Source: CAD feature listing. Evaluate the final solid. Frame: model axes, mm. Face numbers are marked on the shaded views. A direction names the side the tool comes from. Give positions to 0.01 mm unless a question says otherwise; leave off trailing zeros. Order: outer loops, then holes, each group sorted by start corner. A loop starts at its lowest first (then second) coordinate and runs counter-clockwise, first axis right, second up. Notation, with made-up numbers: M 57,-34.5 L 102,-34.5 A33 ccw 102,-3.5 Z; hole C 23,24.5 d2. An arc over 180 degrees is marked long. Answer in a Markdown table with one row per item. Add a question column.
(1) Section query A-A, the plane z = 22. Return loops of the section in (x, y).
(2) Section query C-C, the plane x = 0. Return loops of the section in (y, z), plus the area to 4 significant figures.
(3) Section query B-B, the plane z = 0. Return loops of the section in (x, y).
(4) Material intervals for line 1 along Z through (x, y) = (22, 0.65); line 2 along X through (y, z) = (7.5, 0), sorted ascending.
(5) Pin query (flat end, axial travel): P1, Ø1, axis at y = 2.5, z = -11.5, coming from the -X side; P2, Ø2, axis at y = -0.5, z = -17.5, coming from the +X side. Return the tip coordinate at first contact, or that it passes through.
(6) Section query D-D, the plane x = -22. Return loops of the section in (y, z), plus the area to 3 significant figures.
(7) Set-up query: the marked faces 1 and 2. Return all of +Z, -Z, +X, -X, +Y, -Y with unobstructed straight access to the full face (end or side cutting, diameter ignored); none if empty.
from build123d import *

# Parameters (mm, degrees)
SKETCH1_R                = 27.5
SKETCH1_R_2              = 12.5
SKETCH1_R_3              = 1
BOSS_EXTRUDE1_DEPTH      = 1.5
SKETCH2_R                = 17
SKETCH2_R_2              = 14
BOSS_EXTRUDE2_DEPTH      = 8
CHAMFER1_SIZE            = 0.5
M4_CLEARANCE_HOLE1_D     = 4.5
M4_CLEARANCE_HOLE1_DEPTH = 11.5
M4_CLEARANCE_HOLE1_TIP   = 1.351936393


with BuildPart() as part:
    # Sketch1 → Boss-Extrude1 (new, symmetric)
    with BuildSketch(Plane(origin=(0, 0, 0), x_dir=(1, 0, 0), z_dir=(0, 1, 0))):
        with Locations(Location((0, 0, 0), (0, 0, 270))):
            Circle(SKETCH1_R)
        with Locations(Location((0, 0, 0), (0, 0, 270))):
            Circle(SKETCH1_R_2, mode=Mode.SUBTRACT)
        with Locations(Location((0, 22, 0), (0, 0, 270))):
            Circle(SKETCH1_R_3, mode=Mode.SUBTRACT)
        with Locations(Location((22, 0, 0), (0, 0, 270))):
            Circle(SKETCH1_R_3, mode=Mode.SUBTRACT)
        with Locations(Location((0, -22, 0), (0, 0, 270))):
            Circle(SKETCH1_R_3, mode=Mode.SUBTRACT)
        with Locations(Location((-22, 0, 0), (0, 0, 270))):
            Circle(SKETCH1_R_3, mode=Mode.SUBTRACT)
    extrude(amount=BOSS_EXTRUDE1_DEPTH, both=True)

    # Sketch2 → Boss-Extrude2 (add)
    with BuildSketch(Plane(origin=(0, 1.5, 0), x_dir=(1, 0, 0), z_dir=(0, 1, 0))):
        with Locations(Location((0, 0, 0), (0, 0, 270))):
            Circle(SKETCH2_R)
        with Locations(Location((0, 0, 0), (0, 0, 270))):
            Circle(SKETCH2_R_2, mode=Mode.SUBTRACT)
    extrude(amount=BOSS_EXTRUDE2_DEPTH)

    # Chamfer1
    chamfer1_edges = [part.edges().sort_by_distance(p)[0] for p in [
        (0, 9.5, -17),
        (0, 9.5, -14),
    ]]
    chamfer(chamfer1_edges, length=CHAMFER1_SIZE)

    # M4 Clearance Hole1
    with Locations(Plane(origin=(0, 1.5, 0), x_dir=(1, 0, 0), z_dir=(0, 1, 0))):
        with Locations((0, 22), (22, 0), (-22, 0), (0, -22)):
            Hole(M4_CLEARANCE_HOLE1_D / 2, depth=M4_CLEARANCE_HOLE1_DEPTH)
            with Locations((0, 0, -(M4_CLEARANCE_HOLE1_DEPTH + M4_CLEARANCE_HOLE1_TIP / 2))):  # 118° drill point
                Cone(0, M4_CLEARANCE_HOLE1_D / 2, M4_CLEARANCE_HOLE1_TIP, mode=Mode.SUBTRACT)


solid = part.part
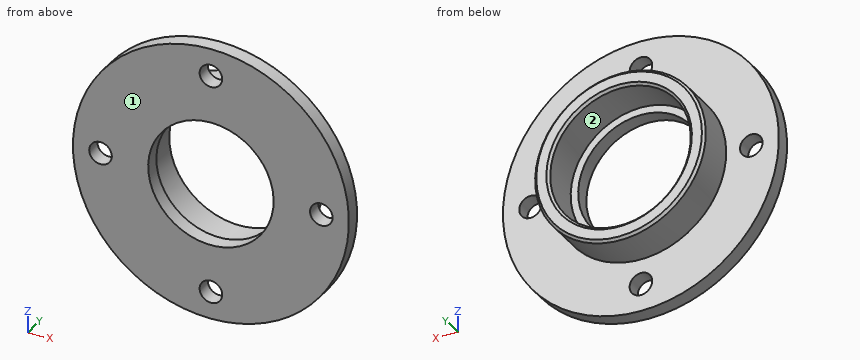
Values follow:
| question | item | result |
|---|---|---|
| 1 | outline | M -16.5,-1.5 L -2.25,-1.5 L -2.25,1.5 L -16.5,1.5 Z; M 2.25,-1.5 L 16.5,-1.5 L 16.5,1.5 L 2.25,1.5 Z |
| 2 | outline | M -1.5,-27.5 L 1.5,-27.5 L 1.5,-24.25 L -1.5,-24.25 Z; M -1.5,-19.75 L 1.5,-19.75 L 1.5,-17 L 9,-17 L 9.5,-16.5 L 9.5,-14.5 L 9,-14 L 1.5,-14 L 1.5,-12.5 L -1.5,-12.5 Z; M -1.5,12.5 L 1.5,12.5 L 1.5,14 L 9,14 L 9.5,14.5 L 9.5,16.5 L 9,17 L 1.5,17 L 1.5,19.75 L -1.5,19.75 Z; M -1.5,24.25 L 1.5,24.25 L 1.5,27.5 L -1.5,27.5 Z |
| 2 | area | 110.5 mm² |
| 3 | outline | M -27.5,-1.5 L -24.25,-1.5 L -24.25,1.5 L -27.5,1.5 Z; M -19.75,-1.5 L -12.5,-1.5 L -12.5,1.5 L -14,1.5 L -14,9 L -14.5,9.5 L -16.5,9.5 L -17,9 L -17,1.5 L -19.75,1.5 Z; M 12.5,-1.5 L 19.75,-1.5 L 19.75,1.5 L 17,1.5 L 17,9 L 16.5,9.5 L 14.5,9.5 L 14,9 L 14,1.5 L 12.5,1.5 Z; M 24.25,-1.5 L 27.5,-1.5 L 27.5,1.5 L 24.25,1.5 Z |
| 4 | line 1 | z = -16.5 to -2.25, 2.25 to 16.5 |
| 4 | line 2 | x = -17 to -14, 14 to 17 |
| 5 | P1 | stops at x = -12.96 |
| 5 | P2 | stops at x = 22 |
| 6 | outline | M -1.5,-16.5 L 1.5,-16.5 L 1.5,-2.25 L -1.5,-2.25 Z; M -1.5,2.25 L 1.5,2.25 L 1.5,16.5 L -1.5,16.5 Z |
| 6 | area | 85.5 mm² |
| 7 | face 1 | +Z, -Z, +X, -X, -Y |
| 7 | face 2 | +Y |
